Geometry: final body of the model. Coordinates: model frame, mm. A direction names the side the tool comes from. Give positions to 0.01 mm unless a question says otherwise; leave off trailing zeros. Order: outer loops, then holes, each group sorted by start corner. A loop starts at its lowest first (then second) coordinate and runs counter-clockwise, first axis right, second up. Notation, with made-up numbers: (14, -30) -> (70, -30) arc R25 cw to (70, -6) -> close; hole circle Ø2 at (63, 14). An arc over 180 degrees is marked (long way). One line per item, written item: value. Start each with the question number.
```python
from build123d import *

# Parameters (mm, degrees)
F2_DEPTH = 19.05
F1_R     = 38.9599032657
F3_DEPTH = 6.35
F4_D     = 6.35


with BuildPart() as f2:
    # F0 (on Top) → F2 (new body)
    with BuildSketch(Plane.XY):
        Polygon((-46.7784367502, 32.4274450541), (-57.2518631816, 32.4274450541), (-71.9749704003, -7.0572411641), (-62.3826421797, -7.0572411641), (-56.3522954025, 9.1150482002), (-56.3522954025, -7.0572411641), (-47.213383019, -7.0572411641), (-32.4902758002, 32.4274450541), (-41.4133742452, 32.4274450541), (-48.040356487, 15.5276963487), align=None)
    extrude(amount=F2_DEPTH)



with BuildPart() as f2b:
    # F0 (on Top) → F2, piece 2 (new body)
    with BuildSketch(Plane.XY):
        Polygon((-35.947676748, -7.1813631803), (-21.5117447078, 32.7009521425), (-30.4481759667, 32.7009521425), (-45.2453941107, -7.0572411641), align=None)
    extrude(amount=F2_DEPTH)


with BuildPart() as f2c:
    # F0 (on Top) → F2, piece 3 (new body)
    with BuildSketch(Plane.XY):
        with BuildLine():
            Line((-14.9974728457, 20.7705546892), (-10.6590073556, 32.4274450541))
            Line((-10.6590073556, 32.4274450541), (-19.8539756238, 32.7009521425))
            Line((-19.8539756238, 32.7009521425), (-34.6973895427, -7.1813631803))
            Line((-34.6973895427, -7.1813631803), (-25.0511299819, -7.1813631803))
            Line((-25.0511299819, -7.1813631803), (-19.1294675285, 8.7293707311))
            Line((-19.1294675285, 8.7293707311), (-19.1294675285, -7.1813631803))
            Line((-19.1294675285, -7.1813631803), (-5.8616320603, -7.1813631803))
            Line((-5.8616320603, -7.1813631803), (-55.7639412582, -20.8262596279))
            ThreePointArc((-55.7639412582, -20.8262596279), (-63.4022025331, -21.3981451994), (-70.6976205111, -19.0642718226))
            ThreePointArc((-70.6976205111, -19.0642718226), (-74.472426735, -15.5960277609), (-76.4715448022, -10.8757093549))
            ThreePointArc((-76.4715448022, -10.8757093549), (-76.1562173184, -2.0282490142), (-72.7623030543, 6.14844542))
            ThreePointArc((-72.7623030543, 6.14844542), (-85.358680949, -10.9955429484), (-91.9176340103, -31.233260408))
            ThreePointArc((-91.9176340103, -31.233260408), (-89.2652472877, -37.3547894918), (-84.1291844845, -41.6126213968))
            ThreePointArc((-84.1291844845, -41.6126213968), (-72.2500160336, -44.1096014144), (-60.3708475828, -41.6126213968))
            Line((-60.3708475828, -41.6126213968), (54.6953529119, 8.9968936518))
            Line((54.6953529119, 8.9968936518), (12.0426900685, -2.3953781929))
            Line((12.0426900685, -2.3953781929), (12.5787025318, 0.2347060363))
            Line((12.5787025318, 0.2347060363), (1.8387236853, 0.2347060363))
            Line((1.8387236853, 0.2347060363), (5.5321310647, 10.158409473))
            Line((5.5321310647, 10.158409473), (14.3720662783, 10.158409473))
            Line((14.3720662783, 10.158409473), (17.1257853508, 17.5572931099))
            Line((17.1257853508, 17.5572931099), (8.5047732013, 17.5572931099))
            Line((8.5047732013, 17.5572931099), (11.5288449451, 25.6825790789))
            Line((11.5288449451, 25.6825790789), (20.8120857023, 25.6825790789))
            Line((20.8120857023, 25.6825790789), (23.3223922551, 32.4274450541))
            Line((23.3223922551, 32.4274450541), (-5.8616320603, 32.4274450541))
            Line((-5.8616320603, 32.4274450541), (-14.9974728457, 20.7705546892))
        make_face()
        Polygon((3.4076007732, 30.4201329794), (-9.3637462705, -3.8948091678), (-9.8301135004, 16.0215999931), align=None, mode=Mode.SUBTRACT)
    extrude(amount=F2_DEPTH)


with BuildPart() as f2_1:
    add(f2.part)

    add(f2b.part)  # F3 merges F2b

    add(f2c.part)  # F3 merges F2c
    # F1 (on Top) → F3 (join)
    with BuildSketch(Plane.XY):
        with Locations((-26.0827448219, 13.5601842776)):
            Circle(F1_R)
    extrude(amount=F3_DEPTH)

    # F4 (through all)
    with Locations(Plane(origin=(0, 0, 0), x_dir=(1, 0, 0), z_dir=(0, 0, -1))):
        with Locations((-26.6133137047, -42.7415519953)):
            Hole(F4_D / 2)


solid = f2_1.part
```
1. Cut plane A-A, the plane z = 4.25. Return loops of the section in (x, y) (3 decimals), then the cut area to 3 significant figures.
2. Draft query along Y for faces 5 (the flat face through (11, 20, 6.35)), 6 (the cylindrical face through (-72.42, -44.11, 9.39)), 7 (the flat face through (9, 32.427, 12)). Return one class per face: pulls with the +Y half, pulls with the -Y half, needs draft (parallel to the pull), parting line crosses it, or undercut.
3. Access query for faces 1 (the cylindrical face through (12.125, 21.178, 3.131)), 2 (the flat face through (-53, 13, 19.05)), 3 (the flat face through (3.66, 5.13, 12.61)), 4 (the flat face through (13, 17.557, 12)). Directions: +Z, -Z, +X, -X, +Y, -Y. A direction counts if a zero-diameter tool reaches every point of the face in a straight line with its end or side. Return the directions, or none.
4. Material intervals for L1, parallel to X at y = 14, z = 11.5; L2, parallel to X at y = 20.5, z = 12.25; L3, parallel to Y at x = 19, z = 17.25, sorted ascending. Write a range as [from, to].
5. Pin query (flat end, axial travel): P1, Ø2, axis at y = -20.5, z = 3.5, coming from the +X side; P2, Ø4, axis at y = 34.5, z = 7, coming from the -X side; P3, Ø4, axis at y = 3, z = 10, coming from the -X side. Return the tip coordinate at first contact, or that it passes through.
6. Cut plane B-B, the plane x = -68. Return loops of the section in (y, z), then the cut area to 3 significant figures.
7. Cut plane D-D, the plane x = -4. Return loops of the section in (y, z), then the cut area to 3 significant figures.
8. Cut plane C-C, the plane z = 13.25. State how many separate pieces and enclosed holes the cut face has, then the cut area to 3 significant figures.
Answers follow:
1. outline: (-91.918, -31.233) arc R14.334 ccw to (-84.129, -41.613) arc R29.506 ccw to (-60.371, -41.613) -> (-23.279, -25.299) arc R38.96 ccw to (0.665, -14.767) -> (54.695, 8.997) -> (12.043, -2.395) -> (12.579, 0.235) -> (10.527, 0.235) arc R38.96 ccw to (12.728, 10.158) -> (14.372, 10.158) -> (17.126, 17.557) -> (12.672, 17.557) arc R38.96 ccw to (11.212, 24.83) -> (11.529, 25.683) -> (20.812, 25.683) -> (23.322, 32.427) -> (8.004, 32.427) arc R38.96 ccw to (-64.996, 11.659) -> (-71.975, -7.057) -> (-62.383, -7.057) -> (-61.079, -3.561) arc R38.96 ccw to (-47.944, -18.688) -> (-55.764, -20.826) arc R20.052 cw to (-70.698, -19.064) arc R12.094 cw to (-76.472, -10.876) arc R24.875 cw to (-72.762, 6.148) arc R66.714 ccw to start; hole circle Ø6.35 at (-26.613, 42.742)
1. area: 6,430 mm²
2. face 5: undercut
2. face 6: pulls with the -Y half
2. face 7: pulls with the +Y half
3. face 1: +Z, -Z, +X
3. face 2: +Z, +X, -X, +Y, -Y
3. face 3: +Z
3. face 4: +Z, +X
4. L1: x = [-64.12, -39.36], [-37.41, -28.28], [-26.81, -9.78], [-2.7, 15.8]
4. L2: x = [-61.7, -47.67], [-46.09, -36.94], [-34.99, -25.93], [-24.39, -5.71], [-0.28, 9.6]
4. L3: y = [-6.7, -0.54], [25.68, 32.43]
5. P1: stops at x = -5.47
5. P2: stops at x = -60.07
5. P3: stops at x = -77.48
6. outline: (-43.8, 0) -> (-20.29, 0) -> (-20.29, 19.05) -> (-43.8, 19.05) -> close; (-7.06, 0) -> (3.6, 0) -> (3.6, 19.05) -> (-7.06, 19.05) -> close
6. area: 651 mm²
7. outline: (-18.54, 0) -> (45.66, 0) -> (45.66, 6.35) -> (32.43, 6.35) -> (32.43, 19.05) -> (22.36, 19.05) -> (22.36, 6.35) -> (10.52, 6.35) -> (10.52, 19.05) -> (-16.82, 19.05) -> (-16.82, 6.35) -> (-18.54, 6.35) -> close
7. area: 883 mm²
8. separate pieces: 3
8. enclosed holes: 1
8. area: 4,550 mm²
